Work out the finished part from the listing and answer in its coordinate system (mm). A direction names the side the tool comes from. Give positions to 0.01 mm unless a question says otherwise; leave off trailing zeros. Loops run counter-clockwise (first coordinate to the right, second up) from the corner with the lowest first, then second, coordinate; pieces in that order, holes last. Notation, with made-up numbers: (85, -34.75) - (101, -34.75) arc R25 cw to (101, -14.75) - close; hole circle Ø8 at (7.5, 77). An arc over 180 degrees is marked (long way). One line per item, written item: value.
from build123d import *

# Parameters (mm, degrees)
F0_W     = 48.9477626979
F0_H     = 23.0111181736
F1_DEPTH = 12.7
F3_DEPTH = 36.83
F4_W     = 30.2896779031
F4_H     = 32.1149742231
F5_DEPTH = 0.5
F5_TAPER = -40


# Not quite as in the source:
# - the program builds the solid bodies; features that only make, move or delete a surface that nothing else refers to are left out


with BuildPart() as f1:
    # F0 (on Top) → F1 (new body)
    with BuildSketch(Plane.XY):
        with Locations((0, -11.5055590868)):
            Rectangle(F0_W, F0_H)
    extrude(amount=F1_DEPTH)

    # F2 (on face) → F3 (join)
    with BuildSketch(Plane.XZ.offset(23.0111181736)):
        Polygon((29.4724665582, 0), (24.473881349, 12.7), (24.473881349, 0), align=None)
        Polygon((-24.473881349, 0), (-24.473881349, 12.7), (-29.4724665582, 0), align=None)
    extrude(amount=-F3_DEPTH)

    # F4 (on face) → F5 (join)
    with BuildSketch(Plane.XY.offset(12.7)):
        with Locations((-0.0495417044, -18.2598386891)):
            Rectangle(F4_W, F4_H)
    extrude(amount=F5_DEPTH, taper=F5_TAPER)


solid = f1.part
1. Flat-ended cylindrical pins translate along their axes: pin 1 Ø3.5 at (x, y) = (3, -28) entering from -Z; pin 2 Ø1 at (x, y) = (-18.5, -7) entering from +Z; pin 3 Ø1 at (x, z) = (0.5, 4.5) entering from +Y. Find the tip coordinate at first contact, or state that the pin passes through.
Output:
pin 1: stops at z = 12.7
pin 2: stops at z = 12.7
pin 3: stops at y = 0
2. Section A-A (y = 10) is taken. Write down the section's boundary in (x, z).
Output:
outline: (-29.47, 0) - (-24.47, 0) - (-24.47, 12.7) - close; (24.47, 0) - (29.47, 0) - (24.47, 12.7) - close
3. For faces 1 (the flat face through (27.01, -4.85, 6.26)), 2 (the flat face through (24.474, 7, 6)), 3 (the flat face through (0, -29, 12.7)), determine the directions among +Z, -Z, +X, -X, +Y, -Y from which every point of the face is accessible in a straight line to the end or side of a thin tool.
Output:
face 1: +Z, +X, +Y, -Y
face 2: +Z, -Z, +Y
face 3: -Z, +X, -X, -Y
4. Find the intervals of material crossed by line 1 along Z through (x, y) = (-3.5, -32.5); line 2 along Y through (x, z) = (4, 1.5); line 3 along Z through (x, y) = (-22.5, -4), in increasing order.
Output:
line 1: z = 12.7 to 13.2
line 2: y = -23.01 to 0
line 3: z = 0 to 12.7
5. Section D-D (y = -1) is taken. Write down the section's boundary in (x, z).
Output:
outline: (-29.47, 0) - (29.47, 0) - (24.47, 12.7) - (-24.47, 12.7) - close
6. Section B-B (z = 6.75) is taken. Write down the section's boundary in (x, y), and give its area (3 significant figures).
Output:
outline: (-26.82, -23.01) - (26.82, -23.01) - (26.82, 13.82) - (24.47, 13.82) - (24.47, 0) - (-24.47, 0) - (-24.47, 13.82) - (-26.82, 13.82) - close
area: 1,300 mm²
7. Section C-C (x = 22) is taken. Write down the section's boundary in (y, z), and give its area (3 significant figures).
Output:
outline: (-23.01, 0) - (0, 0) - (0, 12.7) - (-23.01, 12.7) - close
area: 292 mm²
